Part model, mm, in its own coordinate system. A direction names the side the tool comes from. Give positions to 0.01 mm unless a question says otherwise; leave off trailing zeros. Write each loop counter-clockwise with the first axis right and the second up, starting at its lowest first coordinate (ties: lowest second). Pieces come first, ordered by that corner, then holes. Notation, with made-up numbers: M -3,20 L 27,20 A9 ccw 27,34 Z; hole C -14,64 d2. An arc over 180 degrees is marked long. Answer as CSV lines item,"result". Start each with the question number.
1) Slice it at D-D, the plane x = 0. Give the cut face in (y, z), plus the area to 3 significant figures.
2) Mould opens along X. For faces 4 (the flat face through (-10.4, -2.7, 16)), 5 (the flat face through (-1.5, 6, 12)), 6 (the flat face through (-6, 7, 8)), 7 (the cylindrical face through (-11.4, -6.93, 5.65)) say: pulls with the +X half, pulls with the -X half, needs draft (parallel to the pull), parting line crosses it, or undercut.
3) Slice it at A-A, the plane z = 9.5. Give the cut face in (x, y).
4) Slice it at B-B, the plane x = 5. Give the cut face in (y, z).
5) Tool access for faces 1 (the flat face through (-2.4, -5.5, 5.8)), 2 (the cylindrical face through (-0.199, 5.785, 26.14)), 3 (the cylindrical face through (4.215, 5.801, 26.14)): list every direction of +Z, -Z, +X, -X, +Y, -Y with a clear straight run to the whole face (end or side of a thin tool).
6) Pin check, flat tips, straight feed: pin 1 Ø5 at (y, z) = (5.5, 19) entering from +X; pin 2 Ø3 at (x, y) = (3.5, 3.5) entering from -Z; pin 3 Ø3 at (y, z) = (0, 18.5) entering from +X; pin 4 Ø2 at (x, y) = (8, 6.5) entering from +Z. Stop position of each tip, or through.
7) Wall check: line 1 along X through (y, z) = (4, 3); line 2 along Y through (x, z) = (9.25, 6.5); line 3 along X through (y, z) = (-6.85, 9.5). Give the ranges that are in metal, low to high. Write a range as from..to.
8) Slice it at C-C, the plane y = -5. Give the cut face in (x, z).
```python
from build123d import *

# Parameters (mm, degrees)
F0_W      = 24
F0_H      = 15
F1_DEPTH  = 16
F2_T      = -2
F4_DEPTH  = 5
F5_W      = 5
F5_H      = 2
F6_DEPTH  = 20
F7_DEPTH  = 5
F9_R      = 0.99999
F10_R     = 2
F11_W     = 8.5
F11_H     = 2
F12_DEPTH = 8
F13_W     = 3.25
F13_H     = 2
F14_DEPTH = 4
F15_DEPTH = 25


# Not quite as in the source:
# - a fillet or chamfer is up to 0.001 mm smaller than in the source, because OpenCascade refuses the exact size


with BuildPart() as f1:
    # F0 (on Top) → F1 (new body)
    with BuildSketch(Plane.XY):
        Rectangle(F0_W, F0_H)
    extrude(amount=F1_DEPTH)

    # F2
    f2_openings = [f1.faces().sort_by_distance(p)[0] for p in [
        (0, 0, 16),
    ]]
    offset(amount=F2_T, openings=f2_openings)

    # F3 (on face) → F4 (cut)
    with BuildSketch(Plane.XZ.offset(7.5)):
        with BuildLine():
            Line((-2, 16), (-2, 13.25))
            ThreePointArc((-2, 13.25), (0, 5.25), (2, 13.25))
            Line((2, 13.25), (2, 16))
            Line((2, 16), (-2, 16))
        make_face()
    extrude(amount=-F4_DEPTH, mode=Mode.SUBTRACT)

    # F5 (on face) → F6 (join)
    with BuildSketch(Plane.XY.offset(16)):
        with Locations((2, 6.5)):
            Rectangle(F5_W, F5_H)
    extrude(amount=F6_DEPTH)

    # F7 (add): a face of the model
    f7_faces = [f1.faces().sort_by_distance(p)[0] for p in [
        (0, 0, 0),
    ]]
    extrude(f7_faces, amount=F7_DEPTH)

    # F9 (radius 1 in the source; OpenCascade refuses exactly that, so slightly less here)
    f9_edges = [f1.edges().sort_by_distance(p)[0] for p in [
        (4.5, 5.5, 26),
        (4.5, 7.5, 26),
        (-0.5, 5.5, 26),
        (-0.5, 7.5, 26),
    ]]
    fillet(f9_edges, radius=F9_R)

    # F10
    f10_edges = [f1.edges().sort_by_distance(p)[0] for p in [
        (12, -7.5, 5.5),
        (-12, -7.5, 5.5),
        (-12, 7.5, 5.5),
        (12, 7.5, 5.5),
    ]]
    fillet(f10_edges, radius=F10_R)

    # F11 (on face) → F12 (cut)
    with BuildSketch(Plane.XY.offset(16)):
        with Locations((-5.75, 6.5)):
            Rectangle(F11_W, F11_H)
    extrude(amount=-F12_DEPTH, mode=Mode.SUBTRACT)

    # F13 (on face) → F14 (cut)
    with BuildSketch(Plane.XY.offset(16)):
        with Locations((8.375, 6.5)):
            Rectangle(F13_W, F13_H)
    extrude(amount=-F14_DEPTH, mode=Mode.SUBTRACT)

    # F8 (on face) → F15 (cut)
    with BuildSketch(Plane.YZ.offset(12)):
        Polygon((7.5, -0.9807621135), (-7.5, -5), (7.5, -5), align=None)
    extrude(amount=-F15_DEPTH, mode=Mode.SUBTRACT)


solid = f1.part
```
Found:
1,outline,"M -7.5,-5 L 7.5,-0.98 L 7.5,16 L 7.37,16 L 7.37,36 L 5.63,36 L 5.63,16 L 5.5,16 L 5.5,2 L -5.5,2 L -5.5,5.25 L -7.5,5.25 Z"
1,area,"144 mm²"
2,face 4,"needs draft"
2,face 5,"undercut"
2,face 6,"undercut"
2,face 7,"pulls with the -X half"
3,outline,"M -12,-5.5 A2 ccw -10,-7.5 L -4.25,-7.5 L -4.25,-5.5 L -10,-5.5 L -10,7.5 A2 ccw -12,5.5 Z; M -1.5,5.5 L 10,5.5 L 10,-5.5 L 4.25,-5.5 L 4.25,-7.5 L 10,-7.5 A2 ccw 12,-5.5 L 12,5.5 A2 ccw 10,7.5 L -1.5,7.5 Z"
4,outline,"M -7.5,-5 L 7.5,-0.98 L 7.5,16 L 5.5,16 L 5.5,2 L -5.5,2 L -5.5,16 L -7.5,16 Z"
5,face 1,"+Z"
5,face 2,"+Z, -X, -Y"
5,face 3,"+Z, +X, -Y"
6,pin 1,"x = 4.5"
6,pin 2,"z = -2.45"
6,pin 3,"through"
6,pin 4,"z = 12"
7,line 1,"-12..-10, 10..12"
7,line 2,"-7.5..-5.5, 5.5..7.5"
7,line 3,"-11.48..-4.25, 4.25..11.48"
8,outline,"M -12,-4.33 L 12,-4.33 L 12,16 L 10,16 L 10,2 L -10,2 L -10,16 L -12,16 Z"
